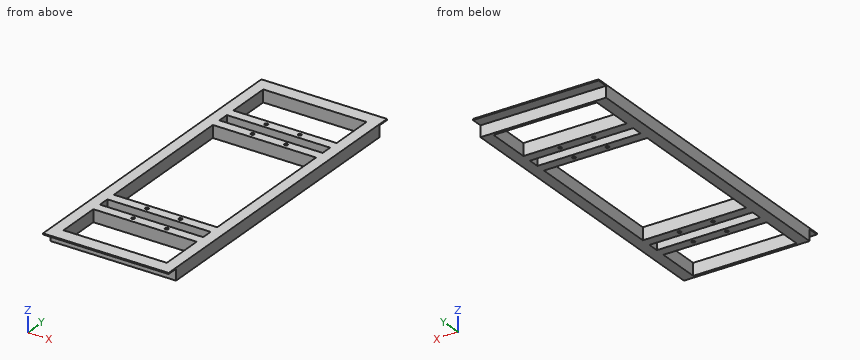
Autodesk Inventor part; units mm, degrees
ref_plane "YZ Plane" through (0, 0, 0) normal (1, 0, 0) x (0, 1, 0)
ref_plane "XZ Plane" through (0, 0, 0) normal (0, 1, 0) x (-1, 0, 0)
ref_plane "XY Plane" through (0, 0, 0) normal (0, 0, 1) x (1, 0, 0)
sketch "草圖1" plane through (0, 0, 0) normal (0, 0, 1) x (1, 0, 0)
  line L0 (0, 0) -> (25, 0)
  line L1 (25.6094, 0) -> (25.6094, 20)
  line L2 (25.6094, 20) -> (250.6094, 20)
  line L3 (250.6094, 20) -> (250.6094, -565)
  line L4 (250.6094, -565) -> (25.6094, -565)
  line L5 (25.6094, -565) -> (25.6094, 20)
  line L6 (25.6094, 0) -> (25.6094, -5)
  line L7 (45.6094, -5) -> (230.6094, -5)
  line L8 (230.6094, -5) -> (230.6094, -85)
  line L9 (230.6094, -85) -> (45.6094, -85)
  line L10 (45.6094, -85) -> (45.6094, -5)
  line L11 (45.6094, -102.5) -> (230.6094, -102.5)
  line L12 (230.6094, -102.5) -> (230.6094, -122.5)
  line L13 (230.6094, -122.5) -> (45.6094, -122.5)
  line L14 (45.6094, -122.5) -> (45.6094, -102.5)
  line L15 (45.6094, -140) -> (230.6094, -140)
  line L16 (230.6094, -140) -> (230.6094, -405)
  line L17 (230.6094, -405) -> (45.6094, -405)
  line L18 (45.6094, -405) -> (45.6094, -140)
  line L19 (45.6094, -422.5) -> (230.6094, -422.5)
  line L20 (230.6094, -422.5) -> (230.6094, -442.5)
  line L21 (230.6094, -442.5) -> (45.6094, -442.5)
  line L22 (45.6094, -442.5) -> (45.6094, -422.5)
  line L23 (45.6094, -460) -> (230.6094, -460)
  line L24 (230.6094, -460) -> (230.6094, -540)
  line L25 (230.6094, -540) -> (45.6094, -540)
  line L26 (45.6094, -540) -> (45.6094, -460)
  dimension "d0" = 25
  dimension "d1" = 20
  dimension "d2" = 225
  dimension "d3" = 585
  dimension "d4" = 5
  dimension "d6" = 20
  dimension "d9" = 185
  dimension "d10" = 80
  dimension "d11" = 185
  dimension "d13" = 185
  dimension "d14" = 20
  dimension "d16" = 185
  dimension "d17" = 265
  dimension "d19" = 185
  dimension "d20" = 20
  dimension "d22" = 185
  dimension "d23" = 80
extrude "擠出1" add sketch "草圖1" along normal blind 2
sketch "草圖2" plane through (0, 0, 0) normal (0, 0, -1) x (-1, 0, 0)
  line L0 (-250.6094, -565) -> (-250.6094, 20)
  line L1 (-250.6094, -565) -> (-250.6094, -545)
  line L2 (-25.6094, 20) -> (-25.6094, -565)
  line L3 (-250.6094, -545) -> (-25.6094, -545)
  line L4 (-25.6094, -545) -> (-25.6094, 0)
  line L5 (-25.6094, 0) -> (-250.6094, 0)
  line L6 (-250.6094, 0) -> (-250.6094, -545)
  line L7 (-230.6094, -460) -> (-230.6094, -540)
  line L8 (-45.6094, -540) -> (-45.6094, -460)
  line L9 (-230.6094, -540) -> (-45.6094, -540)
  line L10 (-45.6094, -540) -> (-45.6094, -460)
  line L11 (-45.6094, -460) -> (-230.6094, -460)
  line L12 (-230.6094, -460) -> (-230.6094, -540)
  line L13 (-230.6094, -442.5) -> (-45.6094, -442.5)
  line L14 (-230.6094, -442.5) -> (-45.6094, -442.5)
  line L15 (-45.6094, -442.5) -> (-45.6094, -422.5)
  line L16 (-45.6094, -422.5) -> (-230.6094, -422.5)
  line L17 (-230.6094, -422.5) -> (-230.6094, -442.5)
  line L18 (-230.6094, -405) -> (-45.6094, -405)
  line L19 (-230.6094, -405) -> (-45.6094, -405)
  line L20 (-45.6094, -405) -> (-45.6094, -140)
  line L21 (-45.6094, -140) -> (-230.6094, -140)
  line L22 (-230.6094, -140) -> (-230.6094, -405)
  line L23 (-230.6094, -122.5) -> (-45.6094, -122.5)
  line L24 (-45.6094, -102.5) -> (-230.6094, -102.5)
  line L25 (-230.6094, -122.5) -> (-45.6094, -122.5)
  line L26 (-45.6094, -122.5) -> (-45.6094, -102.5)
  line L27 (-45.6094, -102.5) -> (-230.6094, -102.5)
  line L28 (-230.6094, -102.5) -> (-230.6094, -122.5)
  line L29 (-230.6094, -85) -> (-45.6094, -85)
  line L30 (-45.6094, -5) -> (-230.6094, -5)
  line L31 (-230.6094, -85) -> (-45.6094, -85)
  line L32 (-45.6094, -85) -> (-45.6094, -5)
  line L33 (-45.6094, -5) -> (-230.6094, -5)
  line L34 (-230.6094, -5) -> (-230.6094, -85)
  circle A0 centre (-25.6094, -102.5) radius 8.75
  line L35 (-25.6094, 20) -> (-25.6094, -565)
  circle A1 centre (-25.6094, -93.75) radius 85
  circle A2 centre (-25.6094, -93.75) radius 145
  circle A3 centre (-170.6094, -93.75) radius 3
  circle A4 centre (-110.6094, -93.75) radius 3
  line L36 (-170.6094, -93.75) -> (-170.6094, -130.75)
  line L37 (-110.6094, -93.75) -> (-110.6094, -130.75)
  circle A5 centre (-110.6094, -130.75) radius 3
  circle A6 centre (-170.6094, -130.75) radius 3
  circle A7 centre (-25.6094, -422.5) radius 8.75
  circle A8 centre (-25.6094, -413.75) radius 85
  circle A9 centre (-25.6094, -413.75) radius 145
  circle A10 centre (-170.6094, -413.75) radius 3
  circle A11 centre (-110.6094, -413.75) radius 3
  line L38 (-110.6094, -413.75) -> (-110.6094, -450.75)
  line L39 (-170.6094, -413.75) -> (-170.6094, -450.75)
  circle A12 centre (-170.6094, -450.75) radius 3
  circle A13 centre (-110.6094, -450.75) radius 3
  point P0 (0, 0)
  dimension "d33" = 17.5
  dimension "d34" = 170
  dimension "d35" = 290
  dimension "d42" = 17.5
  dimension "d43" = 170
  dimension "d44" = 290
  dimension "d26" = 20
  dimension "d27" = 185
  dimension "d28" = 20
  dimension "d29" = 185
  dimension "d30" = 265
  dimension "d36" = 6
  dimension "d37" = 6
  dimension "d38" = 37
  dimension "d39" = 37
  dimension "d40" = 6
  dimension "d41" = 6
  dimension "d45" = 6
  dimension "d46" = 6
  dimension "d47" = 37
  dimension "d48" = 6
  dimension "d49" = 6
extrude "擠出2" add sketch "草圖2" along normal blind 20 contours A12 | A6 | L0 L5 A2 L30 L34 L29 A3 L36 L24 L28 L23 L21 L22 L18 A9 A10 L39 L16 L17 L13 L11 L7 L9 L3 | A9 L9 L8 A8 L2 L3 | L5 L2 A1 L32 L30 A2 | A8 L8 L11 L13 L15 L16 A11 L18 L20 L2 A7 | A13 | A9 L13 A8 L11 | L2 A0 A1 L20 L21 L23 L26 L24 A4 L29 L32 | A2 L20 A1 L2 | L2 A9 L20 A2 | L29 A1 A4 L37 L24 A2 A3 | A7 L2 | L2 A8 L20 A9 | L2 A0 | A3 A2 | A2 L36 A3 | A9 A10 L18 A8 A11 L38 L16 | L16 L39 A10 A9 | A5 | A2 L23 A1 L21 | A4 A1 | A1 L37 A4 | A2 A3 L36 | A3 A2 L24 L36 | L16 L38 A11 A8 | A10 L39 A9 | A9 A10 | A1 A4 L37 | A4 A1 L24 L37 | A11 L38 A8 | A8 A11 | A10 A9 L39 | A11 A8 L38 picked at (-27.5435, -424.6832) picked at (-30.39, -103.7836)
extrude "擠出3" cut sketch "草圖2" along normal through all both and the other way through all contours A12 | A6 | A13 | A3 A2 | A2 L36 A3 | A5 | A4 A1 | A1 L37 A4 | A2 A3 L36 | A10 L39 A9 | A9 A10 | A1 A4 L37 | A11 L38 A8 | A8 A11 | A10 A9 L39 | A11 A8 L38
properties part number "DOF10"
The listing builds one solid part. Answer for the finished solid, in the listing's coordinates (mm). Round coordinates to 2 decimals unless told otherwise and drop trailing zeros. Loops run counter-clockwise (first coordinate to the right, second up) from the corner with the lowest first, then second, coordinate; pieces in that order, holes last. Notation, with made-up numbers: (57.5, 32) - (86.5, 32) arc R15 ccw to (86.5, 45) - close; hole circle Ø6 at (63, -6). An arc over 180 degrees is marked (long way). Return JSON: item names as keys, results as strings. Group by question number.
1. The part is cut by section C-C on z = -10. State how many separate pieces and enclosed holes the cut face has, then the cut area to 3 significant figures.
2. The part is cut by section B-B on x = 143. Determine the outline of the cut face in (y, z), then the cut area to 3 significant figures.
3. The part is cut by section A-A on y = -40.5. Determine the outline of the cut face in (x, z).
4. Consider probe 1 along Y at (x, z) = (129, -5); probe 2 along X at (y, z) = (-235, -5.5); probe 3 along X at (y, z) = (-130.75, -3). Determine where each line is inside the solid, lowest interval first.
5. Each of these flat-tipped pins is pushed along its axis until it touches: P1, Ø5, axis at x = 132.5, z = -16, coming from the -Y side; P2, Ø3, axis at x = 184.5, z = -4.5, coming from the +Y side; P3, Ø6, axis at x = 115.5, y = -552, coming from the -Z side. Where does it stop, or does it pass through?
6. The part is cut by section D-D on x = 236.5. Determine the outline of the cut face in (y, z).
Resolved:
{
 "1": {"separate pieces": "1", "enclosed holes": "13", "area": "36,400 mm²"},
 "2": {"outline": "(-565, 0) - (-545, 0) - (-545, -20) - (-540, -20) - (-540, 2) - (-565, 2) - close; (-460, -20) - (-442.5, -20) - (-442.5, 2) - (-460, 2) - close; (-422.5, -20) - (-405, -20) - (-405, 2) - (-422.5, 2) - close; (-140, -20) - (-122.5, -20) - (-122.5, 2) - (-140, 2) - close; (-102.5, -20) - (-85, -20) - (-85, 2) - (-102.5, 2) - close; (-5, -20) - (0, -20) - (0, 0) - (20, 0) - (20, 2) - (-5, 2) - close", "area": "1,840 mm²"},
 "3": {"outline": "(25.61, -20) - (45.61, -20) - (45.61, 2) - (25.61, 2) - close; (230.61, -20) - (250.61, -20) - (250.61, 2) - (230.61, 2) - close"},
 "4": {"probe 1": "y = -545 to -540, -460 to -442.5, -422.5 to -405, -140 to -122.5, -102.5 to -85, -5 to 0", "probe 2": "x = 25.61 to 45.61, 230.61 to 250.61", "probe 3": "x = 25.61 to 107.61, 113.61 to 167.61, 173.61 to 250.61"},
 "5": {"P1": "stops at y = -545", "P2": "stops at y = 0", "P3": "stops at z = 0"},
 "6": {"outline": "(-565, 0) - (-545, 0) - (-545, -20) - (0, -20) - (0, 0) - (20, 0) - (20, 2) - (-565, 2) - close"}
}
